Input: part model. Units: mm. Frame: model coordinates. A direction names the side the tool comes from. Give positions to 0.01 mm unless a question says otherwise; leave off trailing zeros. Loops run counter-clockwise (first coordinate to the right, second up) from the corner with the lowest first, then second, coordinate; pieces in that order, holes last. Notation, with made-up numbers: M 33.5,-4 L 65.5,-4 A18 cw 65.5,28 Z; hole C 79,-4 d9. An arc over 180 degrees is marked long. Answer as a JSON object with one key per item and string values. Group by question number.
1) Section query A-A on x = 0. Return loops of the section in (y, z), plus the area to 3 significant figures.
2) Section query C-C on z = 129. Return loops of the section in (x, y), plus the area to 3 significant figures.
3) Ray query, L1, parallel to Z at x = 5.5, y = 10; L2, parallel to Y at x = 0.5, z = 102; L3, parallel to Z at x = -16, y = -7. Return the intervals inside material, ascending.
4) Draft query along Z for faces 4 (the flat face through (0, 0, 152)), 5 (the cylindrical face through (-2.38, -10.74, 74.96)), 6 (the cylindrical face through (-13.887, -10.648, 0.986)). Return one class per face: +Z half, -Z half, draft (parallel to the pull), parting line (faces both ways), or undercut.
5) First-contact query: P1, Ø4, axis at y = 1, z = 70, coming from the -X side; P2, Ø8, axis at y = 12, z = 118, coming from the +X side; P3, Ø5, axis at y = -2.5, z = 92.5, coming from the +X side. Flat tips, straight axial feed; report the tip coordinate or a pass-through.
6) Access query for faces 1 (the flat face through (0, 0, 0)), 2 (the flat face through (8, 8, 2)), 3 (the cylindrical face through (9.139, 14.334, 150.986)). Directions: +Z, -Z, +X, -X, +Y, -Y. A direction counts if a zero-diameter tool reaches every point of the face in a straight line with its end or side. Return the directions, or none.
from build123d import *

# Parameters (mm, degrees)
ESQUISSE1_R        = 17.5
BOSS_EXTRU_1_DEPTH = 2
ESQUISSE2_R        = 11
BOSS_EXTRU_2_DEPTH = 150
ESQUISSE3_W        = 6
ESQUISSE3_H        = 2


with BuildPart() as part:
    # Esquisse1 → Boss.-Extru.1 (new body)
    with BuildSketch(Plane.XY):
        Circle(ESQUISSE1_R)
    extrude(amount=BOSS_EXTRU_1_DEPTH)

    # Esquisse2 → Boss.-Extru.2 (add)
    with BuildSketch(Plane.XY.offset(2)):
        Circle(ESQUISSE2_R)
    extrude(amount=BOSS_EXTRU_2_DEPTH)

    # Esquisse3 → Révolution1 (revolve)
    with BuildSketch(Plane(origin=(0, 0, 0), x_dir=(1, 0, 0), z_dir=(0, 1, 0))):
        with Locations((14, -151)):
            Rectangle(ESQUISSE3_W, ESQUISSE3_H)
    revolve(axis=Axis((0, 0, 137.220154247), (0, 0, 1)))


solid = part.part
Output:
{
 "1": {"outline": "M -17.5,0 L 17.5,0 L 17.5,2 L 11,2 L 11,150 L 17,150 L 17,152 L -17,152 L -17,150 L -11,150 L -11,2 L -17.5,2 Z", "area": "3,390 mm^2"},
 "2": {"outline": "C 0,0 d22", "area": "380 mm^2"},
 "3": {"L1": "z = 0 to 2, 150 to 152", "L2": "y = -10.99 to 10.99", "L3": "z = 0 to 2"},
 "4": {"face 4": "+Z half", "face 5": "undercut", "face 6": "draft"},
 "5": {"P1": "stops at x = -11", "P2": "stops at x = 7.55", "P3": "stops at x = 11"},
 "6": {"face 1": "-Z, +X, -X, +Y, -Y", "face 2": "none", "face 3": "+Z"}
}
